from build123d import *

# Parameters (mm, degrees)
CROQUIS1_R              = 1.1
SALIENTE_EXTRUIR1_DEPTH = 2.2
CROQUIS2_R              = 3.5
CROQUIS2_R_2            = 2.3
SALIENTE_EXTRUIR2_DEPTH = 3
CROQUIS3_R              = 2.25
CORTAR_EXTRUIR1_DEPTH   = 1


with BuildPart() as part:
    # Croquis1 → Saliente-Extruir1 (new body)
    with BuildSketch(Plane.XY):
        with BuildLine():
            Line((-7, 25), (-7, 0))
            ThreePointArc((-7, 0), (0, -7), (7, 0))
            Line((7, 0), (7, 25))
            ThreePointArc((7, 25), (0, 32), (-7, 25))
        make_face()
        Circle(CROQUIS1_R, mode=Mode.SUBTRACT)
        with BuildLine():
            ThreePointArc((4, 25), (0, 29), (-4, 25))
            ThreePointArc((-4, 25), (0, 21), (4, 25))
        make_face(mode=Mode.SUBTRACT)
    extrude(amount=SALIENTE_EXTRUIR1_DEPTH)

    # Croquis2 → Saliente-Extruir2 (add)
    with BuildSketch(Plane.XY.offset(2.2)):
        Circle(CROQUIS2_R)
        Circle(CROQUIS2_R_2, mode=Mode.SUBTRACT)
    extrude(amount=SALIENTE_EXTRUIR2_DEPTH)

    # Croquis3 → Cortar-Extruir1 (cut)
    with BuildSketch(Plane(origin=(0, 0, 0), x_dir=(-1, 0, 0), z_dir=(0, 0, -1))):
        Circle(CROQUIS3_R)
    extrude(amount=-CORTAR_EXTRUIR1_DEPTH, mode=Mode.SUBTRACT)


solid = part.part
Read the model definition and answer for the solid it produces. Units are mm, in the model's axes. A direction names the side the tool comes from. Round coordinates to 2 decimals unless told otherwise and drop trailing zeros. Loops run counter-clockwise (first coordinate to the right, second up) from the corner with the lowest first, then second, coordinate; pieces in that order, holes last. Notation, with made-up numbers: (64.25, 56.5) - (106.25, 56.5) arc R13 cw to (106.25, 81.5) - close; hole circle Ø10 at (-30, -11.75). An arc over 180 degrees is marked (long way). One line per question, with ' | ' between items. Start each with the question number.
Q1. Section B-B on z = 0.45 is taken. Give the vertices of the cut face in (x, y).
Q2. Section A-A on x = 0 is taken. Give the vertices of the cut face in (y, z), plus the area to 3 significant figures.
Q3. Section C-C on y = 23.5 is taken. Give the vertices of the cut face in (x, z), plus the area to 3 significant figures.
Q4. Section D-D on z = 4 is taken. Give the vertices of the cut face in (x, y).
Q5. Find the intervals of material crossed by L1, parallel to Y at x = 0, z = 0.65; L2, parallel to Y at x = 0, z = 1.75; L3, parallel to Y at x = 0, z = 2.45, in increasing order.
Q6. For a pull along X with two mould halves and no side action, classify faces 4 (the cylindrical face through (0.521, 21.034, 1.085)), 5 (the cylindrical face through (0, -7, 1)), 6 (the flat face through (-7, 13, 1)), 7 (the flat face through (0, 13, 2.2)) as +X half, -X half, draft (parallel to the pull), parting line (faces both ways), or undercut.
Q7. Flat-ended cylindrical pins translate along their axes: pin 1 (2.5 mm diameter, centred on x = 0.5, y = 0.5, fed in from +Z); pin 2 (1.5 mm diameter, centred on x = 1, z = 1.5, fed in from +Y); pin 3 (1.5 mm diameter, centred on x = -5, z = 3, fed in from -Y). Find the tip coordinate at first contact, or state that the pin passes through.
Q8. For faces 1 (the cylindrical face through (0.29, 2.23, 0.49)), 2 (the flat face through (1, 1, 2.2)), 3 (the cylindrical face through (1.05, 0.33, 1.59)), determine the directions among +Z, -Z, +X, -X, +Y, -Y from which every point of the face is accessible in a straight line to the end or side of a thin tool.
Established:
1) outline: (-7, 0) arc R7 ccw to (7, 0) - (7, 25) arc R7 ccw to (-7, 25) - close; hole circle Ø8 at (0, 25); hole circle Ø4.5 at (0, 0)
2) outline: (-7, 0) - (-2.25, 0) - (-2.25, 1) - (-1.1, 1) - (-1.1, 2.2) - (-2.3, 2.2) - (-2.3, 5.2) - (-3.5, 5.2) - (-3.5, 2.2) - (-7, 2.2) - close; (1.1, 1) - (2.25, 1) - (2.25, 0) - (21, 0) - (21, 2.2) - (3.5, 2.2) - (3.5, 5.2) - (2.3, 5.2) - (2.3, 2.2) - (1.1, 2.2) - close; (29, 0) - (32, 0) - (32, 2.2) - (29, 2.2) - close | area: 68.3 mm²
3) outline: (-7, 0) - (-3.71, 0) - (-3.71, 2.2) - (-7, 2.2) - close; (3.71, 0) - (7, 0) - (7, 2.2) - (3.71, 2.2) - close | area: 14.5 mm²
4) outline: circle Ø7 at (0, 0); hole circle Ø4.6 at (0, 0)
5) L1: -7 to -2.25, 2.25 to 21, 29 to 32 | L2: -7 to -1.1, 1.1 to 21, 29 to 32 | L3: -3.5 to -2.3, 2.3 to 3.5
6) face 4: undercut | face 5: parting line | face 6: -X half | face 7: draft
7) pin 1: z = 2.2 | pin 2: y = 32 | pin 3: through
8) face 1: -Z | face 2: +Z | face 3: +Z, -Z
